```python
from build123d import *

# Parameters (mm, degrees)
F0_R     = 2.7559
F1_DEPTH = 3.175


with BuildPart() as f1:
    # F0 (on Front) → F1 (new body)
    with BuildSketch(Plane.XZ):
        Polygon((-70, 0), (0, 0), (0, 40), (-25, 70), (-45, 70), (-70, 40), align=None)
        with Locations((-52.5, 10.000005)):
            Circle(F0_R, mode=Mode.SUBTRACT)
        with Locations((-52.5, 30.000005)):
            Circle(F0_R, mode=Mode.SUBTRACT)
        with Locations((-17.5, 10.000005)):
            Circle(F0_R, mode=Mode.SUBTRACT)
        with Locations((-17.5, 30.000005)):
            Circle(F0_R, mode=Mode.SUBTRACT)
        with Locations((-35, 47.164548)):
            Circle(F0_R, mode=Mode.SUBTRACT)
        with Locations((-35, 63.27837)):
            Circle(F0_R, mode=Mode.SUBTRACT)
    extrude(amount=-F1_DEPTH)


solid = f1.part
```
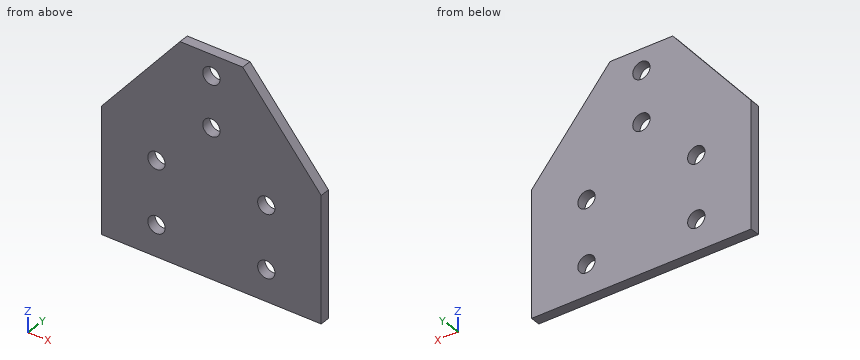
For this review, take the finished solid that the model builds, in its own axes (mm). Coordinates: 2 decimals unless noted, no trailing zeros. Write each loop counter-clockwise with the first axis right and the second up, starting at its lowest first coordinate (ties: lowest second). Pieces come first, ordered by that corner, then holes.
(1) Add section D-D on z = 49. Give the boundary of the cut face in (x, y) (3 decimals).
(2) Add section C-C on x = -35. Give the boundary of the cut face in (y, z) (3 decimals), then the cut area to 3 significant figures.
(3) Add section B-B on y = 1.5. Give the boundary of the cut face in (x, z), then the cut area to 3 significant figures.
(4) Wall thickness on probe 1 along Z at (x, y) = (-35, 1.55); probe 2 along X at (y, z) = (0.6, 32); probe 3 along X at (y, z) = (1.85, 31): over which ranges is each line inside the solid? List them lowest first.
(5) For pin 1 Ø1 at (x, y) = (-46, 2.5) entering from +Z; pin 2 Ø5 at (x, z) = (-52.5, 10) entering from +Y, all flat-tipped, find the tip position at first contact; note any pin that passes through.
(6) Add section A-A on x = -17.5. Give the boundary of the cut face in (y, z) (3 decimals), then the cut area to 3 significant figures.
Answer sheet:
1. outline: (-62.5, 0) - (-37.056, 0) - (-37.056, 3.175) - (-62.5, 3.175) - close; (-32.944, 0) - (-7.5, 0) - (-7.5, 3.175) - (-32.944, 3.175) - close
2. outline: (0, 0) - (3.175, 0) - (3.175, 44.409) - (0, 44.409) - close; (0, 49.92) - (3.175, 49.92) - (3.175, 60.522) - (0, 60.522) - close; (0, 66.034) - (3.175, 66.034) - (3.175, 70) - (0, 70) - close
2. area: 187 mm2
3. outline: (-70, 0) - (0, 0) - (0, 40) - (-25, 70) - (-45, 70) - (-70, 40) - close; hole circle Ø5.51 at (-52.5, 10); hole circle Ø5.51 at (-52.5, 30); hole circle Ø5.51 at (-35, 47.16); hole circle Ø5.51 at (-35, 63.28); hole circle Ø5.51 at (-17.5, 10); hole circle Ø5.51 at (-17.5, 30)
3. area: 4,010 mm2
4. probe 1: z = 0 to 44.41, 49.92 to 60.52, 66.03 to 70
4. probe 2: x = -70 to -54.4, -50.6 to -19.4, -15.6 to 0
4. probe 3: x = -70 to -55.07, -49.93 to -20.07, -14.93 to 0
5. pin 1: stops at z = 69.4
5. pin 2: passes through
6. outline: (0, 0) - (3.175, 0) - (3.175, 7.244) - (0, 7.244) - close; (0, 12.756) - (3.175, 12.756) - (3.175, 27.244) - (0, 27.244) - close; (0, 32.756) - (3.175, 32.756) - (3.175, 61) - (0, 61) - close
6. area: 159 mm2
